Geometry check sheet. Reference: the model listing, model coordinates, mm. A direction names the side the tool comes from. Round coordinates to 2 decimals unless told otherwise and drop trailing zeros. Loops run counter-clockwise (first coordinate to the right, second up) from the corner with the lowest first, then second, coordinate; pieces in that order, holes last. Notation, with made-up numbers: M 52,7.25 L 99,7.25 A22 cw 99,41.25 Z; hole C -38.5,48 d8. An arc over 180 degrees is marked long. Answer in a Markdown table with one row per item. Add a question column.
```python
from build123d import *

# Parameters (mm, degrees)
F0_W        = 16.0388723016
F0_H        = 25.0722588971
F0_W_2      = 17.1450078487
F0_W_3      = 20.0946815312
F0_H_2      = 7.0054841926
F1_DEPTH    = 97.79
F2_W        = 83.8691648096
F2_H        = 58.0902062356
F4_DEPTH    = 23.622
F5_W        = 18.6321306974
F5_H        = 57.669268921
F6_DEPTH    = 23.622
F7_T4_DEPTH = 188.3107647097


# Not quite as in the source:
# - a fillet or chamfer that OpenCascade refuses, or shapes differently, is made with other operations: its cross-section is extruded or revolved along the edge and cut away or added


with BuildPart() as f1:
    # F0 (on Front) → F1 (new body)
    with BuildSketch(Plane.XZ):
        with Locations((-84.1579847038, 2.0279032178)):
            Rectangle(F0_W, F0_H)
        with Locations((93.9287915826, 2.0279032178)):
            Rectangle(F0_W_2, F0_H)
        Polygon((85.3562876582, 14.5640326664), (-76.138548553, 14.5640326664), (-76.138548553, -10.5082262307), (11.0612912104, -10.5082262307), (53.2785467803, -10.5082262307), (53.2785467803, -3.5027420381), (53.2785467803, 3.5027421545), (73.3732283115, 3.5027421545), (73.3732283115, -3.5027420381), (73.3732283115, -10.5082262307), (85.3562876582, -10.5082262307), align=None)
        with Locations((63.3258875459, 5.82e-08)):
            Rectangle(F0_W_3, F0_H_2)
        with Locations((63.3258875459, -7.0054841344)):
            Rectangle(F0_W_3, F0_H_2)
    extrude(amount=-F1_DEPTH)

    # F2 (on face) → F4 (join)
    with BuildSketch(Plane(origin=(0, 0, -10.5082262307), x_dir=(1, 0, 0), z_dir=(0, 0, -1))):
        with Locations((60.5667131022, -54.7835994512)):
            Rectangle(F2_W, F2_H)
    extrude(amount=F4_DEPTH)

    # F5 (on face) → F6 (join)
    with BuildSketch(Plane(origin=(0, 0, -10.5082262307), x_dir=(1, 0, 0), z_dir=(0, 0, -1))):
        with Locations((9.3160653487, -54.7836041078)):
            Rectangle(F5_W, F5_H)
    extrude(amount=F6_DEPTH)

    # F7: chamfer of 25.4 on 1 edges, made by hand


with BuildPart() as f7_tool2:
    # F7_s3 → F7_t4 (new body)
    with BuildSketch(Plane.XZ.offset(39.371778247)):
        Polygon((0, -8.7302262307), (25.4, -34.1302262307), (0, -34.1302262307), align=None)
    extrude(amount=-F7_T4_DEPTH)

    split(bisect_by=Plane.XY.offset(-10.5082262307), keep=Keep.BOTTOM)


with BuildPart() as f1_1:
    add(f1.part)

    # F7_t1: cut F7_tool2
    add(f7_tool2.part, mode=Mode.SUBTRACT)


solid = f1_1.part
```
1) Cross-section at A-A, the plane x = 28. Record the boundary of the cut face in (y, z), plus the area to 3 significant figures.
2) Cross-section at B-B, the plane y = 52. Record the boundary of the cut face in (x, z), plus the area to 3 significant figures.
3) Thickness scan on L1, parallel to Z at x = 74.5, y = 7; L2, parallel to Y at x = 45, z = -15.5; L3, parallel to Y at x = 18.5, z = -22.5. Record the ranges inside material, lowest first. Write a range as [from, to].
4) Go/stop test with flat-tipped pins: pin 1 (5 mm diameter, centred on x = 7.5, z = -17.5, fed in from +Y); pin 2 (7 mm diameter, centred on x = 42, z = -17.5, fed in from -Y); pin 3 (7 mm diameter, centred on x = 76, z = -23, fed in from +Y). Record where each tip stops, or that it passes through.
5) Cross-section at D-D, the plane y = 88.5. Record the boundary of the cut face in (x, z).
6) Cross-section at C-C, the plane x = -36. Record the boundary of the cut face in (y, z), plus the area to 3 significant figures.
7) Set-up check for faces 1 (the flat face through (14, 25.949, -15)), 2 (the flat face through (102.501, 48, -10)), 3 (the flat face through (14, 83.618, -15)), 4 (the flat face through (60, 25.738, -22)), 5 (the flat face through (60, 83.829, -22)): record each of +Z, -Z, +X, -X, +Y, -Y from which the full face is reachable in a straight line by a thin tool's end or side.
Worked answers:
| question | item | result |
|---|---|---|
| 1 | outline | M 0,-10.51 L 25.74,-10.51 L 25.74,-34.13 L 83.83,-34.13 L 83.83,-10.51 L 97.79,-10.51 L 97.79,14.56 L 0,14.56 Z |
| 1 | area | 3,820 mm2 |
| 2 | outline | M -92.18,-10.51 L 1.78,-10.51 L 25.4,-34.13 L 102.5,-34.13 L 102.5,14.56 L -92.18,14.56 Z |
| 2 | area | 6,980 mm2 |
| 3 | L1 | z = [-10.51, 14.56] |
| 3 | L2 | y = [25.74, 83.83] |
| 3 | L3 | y = [25.95, 83.62] |
| 4 | pin 1 | stops at y = 83.62 |
| 4 | pin 2 | stops at y = 25.74 |
| 4 | pin 3 | stops at y = 83.83 |
| 5 | outline | M -92.18,-10.51 L 102.5,-10.51 L 102.5,14.56 L -92.18,14.56 Z |
| 6 | outline | M 0,-10.51 L 97.79,-10.51 L 97.79,14.56 L 0,14.56 Z |
| 6 | area | 2,450 mm2 |
| 7 | face 1 | -Z, -X, -Y |
| 7 | face 2 | +Z, -Z, +X, +Y, -Y |
| 7 | face 3 | -Z, -X, +Y |
| 7 | face 4 | -Z, +X, -X, -Y |
| 7 | face 5 | -Z, +X, -X, +Y |
